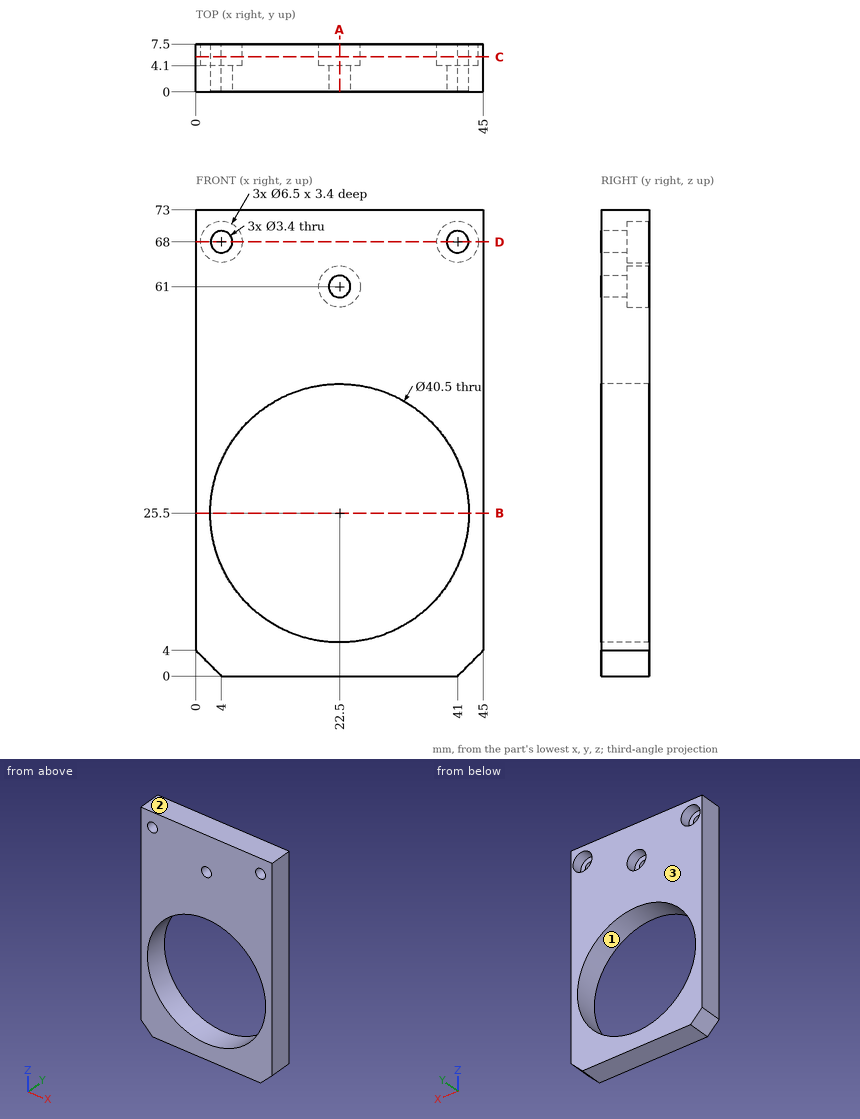
Study the drawing (mm; zero at the part's minimum x, y, z) and answer. Round coordinates to 2 decimals unless told otherwise and drop trailing zeros. Order: outer loops, then holes, each group sorted by start corner. A loop starts at its lowest first (then second) coordinate and runs counter-clockwise, first axis right, second up. Notation, with made-up numbers: (-37, 84) -> (-24, 84) arc R23 ccw to (-24, 107) -> close; hole circle Ø8 at (22.5, 62). An arc over 180 degrees is marked (long way). Answer as CSV lines item,"result". Start each with the question number.
(1) A flat-ended cylindrical pin translates along its axis: pin 1 Ø6 at (x, z) = (22.5, 61) entering from +Y. Find the tip coordinate at first contact, or state that the pin passes through.
(2) For a pull along Z with two mould halves and no side action, classify the marked faces 1, 2 and 3 as +Z half, -Z half, draft (parallel to the pull), parting line (faces both ways), or undercut.
(3) The part is cut by section C-C (y = 5.5). Determine the outline of the cut face in (x, z), then the cut area to 3 significant figures.
(4) The part is cut by section D-D (z = 68). Determine the outline of the cut face in (x, y), then the cut area to 3 significant figures.
(5) Find the intervals of material crossed by probe 1 along Z at (x, y) = (22.5, 4.5); probe 2 along X at (y, z) = (1.8, 68); probe 3 along X at (y, z) = (6.45, 68), in increasing order. Write a range as from..to.
(6) The part is cut by section A-A (x = 22.5). Determine the outline of the cut face in (y, z).
(7) The part is cut by section B-B (z = 25.5). Determine the outline of the cut face in (x, y).
Evaluation:
1,pin 1,"y = 4.1"
2,face 1,"undercut"
2,face 2,"+Z half"
2,face 3,"draft"
3,outline,"(0, 4) -> (4, 0) -> (41, 0) -> (45, 4) -> (45, 73) -> (0, 73) -> close; hole circle Ø6.5 at (4, 68); hole circle Ø40.5 at (22.5, 25.5); hole circle Ø6.5 at (22.5, 61); hole circle Ø6.5 at (41, 68)"
3,area,"1,880 mm²"
4,outline,"(0, 0) -> (2.3, 0) -> (2.3, 4.1) -> (0.75, 4.1) -> (0.75, 7.5) -> (0, 7.5) -> close; (5.7, 0) -> (39.3, 0) -> (39.3, 4.1) -> (37.75, 4.1) -> (37.75, 7.5) -> (7.25, 7.5) -> (7.25, 4.1) -> (5.7, 4.1) -> close; (42.7, 0) -> (45, 0) -> (45, 7.5) -> (44.25, 7.5) -> (44.25, 4.1) -> (42.7, 4.1) -> close"
4,area,"265 mm²"
5,probe 1,"0..5.25, 45.75..57.75, 64.25..73"
5,probe 2,"0..2.3, 5.7..39.3, 42.7..45"
5,probe 3,"0..0.75, 7.25..37.75, 44.25..45"
6,outline,"(0, 0) -> (7.5, 0) -> (7.5, 5.25) -> (0, 5.25) -> close; (0, 45.75) -> (7.5, 45.75) -> (7.5, 57.75) -> (4.1, 57.75) -> (4.1, 59.3) -> (0, 59.3) -> close; (0, 62.7) -> (4.1, 62.7) -> (4.1, 64.25) -> (7.5, 64.25) -> (7.5, 73) -> (0, 73) -> close"
7,outline,"(0, 0) -> (2.25, 0) -> (2.25, 7.5) -> (0, 7.5) -> close; (42.75, 0) -> (45, 0) -> (45, 7.5) -> (42.75, 7.5) -> close"
